Part model, mm, in its own coordinate system. Face numbers are marked on the shaded views. A direction names the side the tool comes from. Give positions to 0.01 mm unless a question says otherwise; leave off trailing zeros. Loops run counter-clockwise (first coordinate to the right, second up) from the corner with the lowest first, then second, coordinate; pieces in that order, holes last. Notation, with made-up numbers: (14, 41.5) -> (26, 41.5) arc R16 ccw to (26, 48.5) -> close; hole circle Ø8 at (14, 13.5). An arc over 180 degrees is marked (long way). Write item = value, one per line.
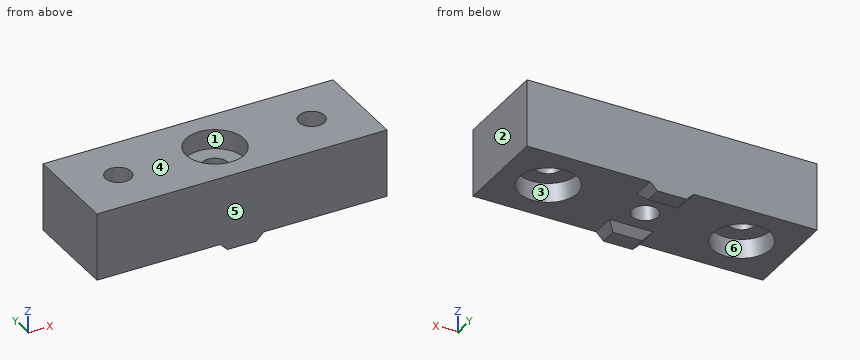
Autodesk Fusion 360 part; units mm, degrees
sketch "Sketch1" plane through (0, 0, 0) normal (0, 0, 1) x (1, 0, 0)
  line L0 (30, -10) -> (-30, -10)
  line L1 (-30, -10) -> (-30, 10)
  line L2 (-30, 10) -> (30, 10)
  line L3 (30, 10) -> (30, -10)
  line L4 (30, -10) -> (-30, 10) construction
  line L5 (-30, -10) -> (30, 10) construction
  circle A0 centre (0, 0) radius 2.65
  circle A1 centre (20, 0) radius 2.65
  circle A2 centre (-20, 0) radius 2.65
  circle A3 centre (-20, 0) radius 6
  circle A4 centre (20, 0) radius 6
  dimension "d1" = 60
  dimension "d2" = 20
  dimension "d3" = 5.3
  dimension "d4" = 5.3
  dimension "d5" = 5.3
  dimension "d11" = 12
  dimension "d12" = 12
extrude "Extrude1" add sketch "Sketch1" along normal blind 6 contours L0 L1 L2 L3 | A3 | A4
sketch "Sketch2" plane through (0, 0, 6) normal (0, 0, 1) x (-1, 0, 0)
  circle A0 centre (0, 0) radius 2.65
  circle A1 centre (-20, 0) radius 2.65
  circle A2 centre (20, 0) radius 2.65
  line L0 (-30, -10) -> (30, -10)
  line L1 (30, -10) -> (30, 10)
  line L2 (30, 10) -> (-30, 10)
  line L3 (-30, 10) -> (-30, -10)
  circle A3 centre (0, 0) radius 6
  dimension "d8" = 12
extrude "Extrude2" add sketch "Sketch2" along normal blind 4 contours L0 L1 L2 L3
extrude "Extrude4" add sketch "Sketch1" against normal blind 4 contours L0 L1 L2 L3
sketch "Sketch3" plane through (0, 0, -4) normal (0, 0, -1) x (1, 0, 0)
  circle A0 centre (0, 0) radius 2.65
  circle A1 centre (20, 0) radius 6
  circle A2 centre (-20, 0) radius 6
  line L0 (-30, -10) -> (30, -10)
  line L1 (30, -10) -> (30, 10)
  line L2 (30, 10) -> (-30, 10)
  line L3 (-30, 10) -> (-30, -10)
  line L4 (-4.5, 5) -> (4.5, 5)
  line L5 (4.5, 5) -> (4.5, 10)
  line L6 (4.5, 10) -> (-4.5, 10)
  line L7 (-4.5, 10) -> (-4.5, 5)
  line L8 (-4.5, -10) -> (4.5, -10)
  line L9 (4.5, -10) -> (4.5, -5)
  line L10 (4.5, -5) -> (-4.5, -5)
  line L11 (-4.5, -5) -> (-4.5, -10)
  dimension "d17" = 9
  dimension "d18" = 5
  dimension "d19" = 9
  dimension "d20" = 5
extrude "Extrude5" add sketch "Sketch3" along normal blind 1.5 contours L0 L8 L9 L10 L11 | L2 L4 L5 L6 L7
chamfer "Chamfer1" distance 1.5 angle 45 6 edges at (-4.5, -7.5, -5.5) (0, -5, -5.5) (4.5, -7.5, -5.5) (-4.5, 7.5, -5.5) (0, 5, -5.5) (4.5, 7.5, -5.5)
extrude "Extrude3" [suppressed]
1) Slice it at C-C, the plane y = 0. List the corners of the cut face in (x, z).
Resolved:
outline = (-30, -4) -> (-26, -4) -> (-26, 0) -> (-22.65, 0) -> (-22.65, 10) -> (-30, 10) -> close; (-17.35, 0) -> (-14, 0) -> (-14, -4) -> (-2.65, -4) -> (-2.65, 6) -> (-6, 6) -> (-6, 10) -> (-17.35, 10) -> close; (2.65, -4) -> (14, -4) -> (14, 0) -> (17.35, 0) -> (17.35, 10) -> (6, 10) -> (6, 6) -> (2.65, 6) -> close; (22.65, 0) -> (26, 0) -> (26, -4) -> (30, -4) -> (30, 10) -> (22.65, 10) -> close
2) Slice it at B-B, the plane z = -2. List the corners of the cut face in (x, y).
Resolved:
outline = (-30, -10) -> (30, -10) -> (30, 10) -> (-30, 10) -> close; hole circle Ø12 at (-20, 0); hole circle Ø5.3 at (0, 0); hole circle Ø12 at (20, 0)
3) Drop flat-ended pins along their axis: P1, Ø7, axis at x = 0, y = 0, coming from the -Z side; P2, Ø7, axis at x = -20, y = 0, coming from the +Z side; P3, Ø9.5, axis at x = 20, y = 0, coming from the -Z side. Give the stop position or say it passes through.
Resolved:
P1 = -4
P2 = 10
P3 = 0
4) Drill centre lines: line 1 along X through (y, z) = (0, 7.9); line 2 along Y through (x, z) = (-20, 5); line 3 along X through (y, z) = (0.25, 3.5). Where is each one in solid material? Low to high. Write a range as [from, to].
Resolved:
line_1 = [-30, -22.65], [-17.35, -6], [6, 17.35], [22.65, 30]
line_2 = [-10, -2.65], [2.65, 10]
line_3 = [-30, -22.64], [-17.36, -2.64], [2.64, 17.36], [22.64, 30]
5) Pull direction Y, two halves, no side cores. Call the marked faces 4, 5 and 6: pulls with the +Y half, pulls with the -Y half, needs draft (parallel to the pull), parting line crosses it, or undercut.
Resolved:
face_4 = needs draft
face_5 = pulls with the -Y half
face_6 = undercut
6) Which spindle directions (+Z, -Z, +X, -X, +Y, -Y) get a long thin tool onto all of the face, cutting with end or side? Do the marked faces 1, 2 and 3. Say none if no direction does.
Resolved:
face_1 = +Z
face_2 = +Z, -Z, +X, +Y, -Y
face_3 = -Z
7) Slice it at D-D, the plane x = -20. List the corners of the cut face in (y, z), and give its area (3 significant figures).
Resolved:
outline = (-10, -4) -> (-6, -4) -> (-6, 0) -> (-2.65, 0) -> (-2.65, 10) -> (-10, 10) -> close; (2.65, 0) -> (6, 0) -> (6, -4) -> (10, -4) -> (10, 10) -> (2.65, 10) -> close
area = 179 mm²
